from build123d import *

# Parameters (mm, degrees)
F0_R         = 12.5
F1_DEPTH     = 3
F2_R         = 4
F3_DEPTH     = 30
F4_W         = 68
F4_H         = 8
F5_DEPTH     = 8
F6_R         = 3.9999
F7_T8_DEPTH  = 60
F7_S9_R      = 4
F7_T10_DEPTH = 32
F7_S11_R     = 4
F7_T12_DEPTH = 32
F7_T16_DEPTH = 60
F7_S17_R     = 4
F7_T18_DEPTH = 32
F7_S19_R     = 4
F7_T20_DEPTH = 32


# Not quite as in the source:
# - a fillet or chamfer that OpenCascade refuses, or shapes differently, is made with other operations: its cross-section is extruded or revolved along the edge and cut away or added
# - two fillets or chamfers of one size are made in one step
# - a fillet or chamfer is up to 0.001 mm smaller than in the source, because OpenCascade refuses the exact size


with BuildPart() as f1:
    # F0 (on Top) → F1 (new body)
    with BuildSketch(Plane.XY):
        with Locations((-30, 0)):
            Circle(F0_R)
    extrude(amount=F1_DEPTH)

    # F2 (on face) → F3 (join)
    with BuildSketch(Plane.XY.offset(3)):
        with Locations((-30, 0)):
            Circle(F2_R)
    extrude(amount=F3_DEPTH)



with BuildPart() as f1b:
    # F0 (on Top) → F1, piece 2 (new body)
    with BuildSketch(Plane.XY):
        with Locations((30, 0)):
            Circle(F0_R)
    extrude(amount=F1_DEPTH)

    # F2 (on face) → F3, piece 2 (join)
    with BuildSketch(Plane.XY.offset(3)):
        with Locations((30, 0)):
            Circle(F2_R)
    extrude(amount=F3_DEPTH)


with BuildPart() as f1_1:
    add(f1.part)

    add(f1b.part)  # F5 merges F1b
    # F4 (on face) → F5 (join)
    with BuildSketch(Plane.XY.offset(33)):
        Rectangle(F4_W, F4_H)
    extrude(amount=-F5_DEPTH)

    # F6 (radius 4 in the source; OpenCascade refuses exactly that, so slightly less here)
    f6_edges = [f1_1.edges().sort_by_distance(p)[0] for p in [
        (34, 0, 33),
        (0, 4, 33),
        (-34, 0, 33),
        (0, -4, 33),
        (34, -4, 29),
        (34, 4, 29),
        (-34, -4, 29),
        (-34, 4, 29),
    ]]
    fillet(f6_edges, radius=F6_R)

    # F7: fillet of radius 3 on 6 edges, made by hand

    # F7_s1 → F7_t2 (revolve)
    with BuildSketch(Plane.XZ):
        with BuildLine():
            ThreePointArc((33.9996, 6.0009656854), (34.8786796564, 3.8786796564), (37.0009656854, 2.9996))
            Line((37.0009656854, 2.9996), (37.0009656854, 2.6994634315))
            ThreePointArc((37.0009656854, 2.6994634315), (35.5004828427, 2.6998634315), (34, 2.6998634315))
            Line((34, 2.6998634315), (33.6998634315, 3))
            ThreePointArc((33.6998634315, 3), (33.6998634315, 4.5004828427), (33.6994634315, 6.0009656854))
            Line((33.6994634315, 6.0009656854), (33.9996, 6.0009656854))
        make_face()
    revolve(axis=Axis((30, 0, 3), (0, 0, 1)))

    # F7_s3 → F7_t4 (revolve)
    with BuildSketch(Plane.XZ):
        with BuildLine():
            ThreePointArc((-26.0004, 6.0009656854), (-25.1213203436, 3.8786796564), (-22.9990343146, 2.9996))
            Line((-22.9990343146, 2.9996), (-22.9990343146, 2.6994634315))
            ThreePointArc((-22.9990343146, 2.6994634315), (-24.4995171573, 2.6998634315), (-26, 2.6998634315))
            Line((-26, 2.6998634315), (-26.3001365685, 3))
            ThreePointArc((-26.3001365685, 3), (-26.3001365685, 4.5004828427), (-26.3005365685, 6.0009656854))
            Line((-26.3005365685, 6.0009656854), (-26.0004, 6.0009656854))
        make_face()
    revolve(axis=Axis((-30, 0, 3), (0, 0, 1)))


with BuildPart() as f7_tool6:
    # F7_s7 → F7_t8 (new body)
    with BuildSketch(Plane.YZ.offset(-30)):
        with BuildLine():
            ThreePointArc((-0.9990343146, 24.9996), (-3.1213203436, 25.8786796564), (-4.0004, 28.0009656854))
            Line((-4.0004, 28.0009656854), (-4.3005365685, 28.0009656854))
            ThreePointArc((-4.3005365685, 28.0009656854), (-4.3001365685, 26.5004828427), (-4.3001365685, 25))
            Line((-4.3001365685, 25), (-4, 24.6998634315))
            ThreePointArc((-4, 24.6998634315), (-2.4995171573, 24.6998634315), (-0.9990343146, 24.6994634315))
            Line((-0.9990343146, 24.6994634315), (-0.9990343146, 24.9996))
        make_face()
    extrude(amount=F7_T8_DEPTH)

    # F7_s9 → F7_t10 (cut, symmetric)
    with BuildSketch(Plane.XY.offset(26.4)):
        with Locations((30, 0)):
            Circle(F7_S9_R)
    extrude(amount=F7_T10_DEPTH, both=True, mode=Mode.SUBTRACT)

    # F7_s11 → F7_t12 (cut, symmetric)
    with BuildSketch(Plane.XY.offset(26.4)):
        with Locations((-30, 0)):
            Circle(F7_S11_R)
    extrude(amount=F7_T12_DEPTH, both=True, mode=Mode.SUBTRACT)


with BuildPart() as f1_2:
    add(f1_1.part)

    # F7_t5: cut F7_tool6
    add(f7_tool6.part, mode=Mode.SUBTRACT)


with BuildPart() as f7_tool14:
    # F7_s15 → F7_t16 (new body)
    with BuildSketch(Plane.YZ.offset(30)):
        with BuildLine():
            ThreePointArc((4.0004, 28.0009656854), (3.1213203436, 25.8786796564), (0.9990343146, 24.9996))
            Line((0.9990343146, 24.9996), (0.9990343146, 24.6994634315))
            ThreePointArc((0.9990343146, 24.6994634315), (2.4995171573, 24.6998634315), (4, 24.6998634315))
            Line((4, 24.6998634315), (4.3001365685, 25))
            ThreePointArc((4.3001365685, 25), (4.3001365685, 26.5004828427), (4.3005365685, 28.0009656854))
            Line((4.3005365685, 28.0009656854), (4.0004, 28.0009656854))
        make_face()
    extrude(amount=-F7_T16_DEPTH)

    # F7_s17 → F7_t18 (cut, symmetric)
    with BuildSketch(Plane.XY.offset(26.4)):
        with Locations((30, 0)):
            Circle(F7_S17_R)
    extrude(amount=F7_T18_DEPTH, both=True, mode=Mode.SUBTRACT)

    # F7_s19 → F7_t20 (cut, symmetric)
    with BuildSketch(Plane.XY.offset(26.4)):
        with Locations((-30, 0)):
            Circle(F7_S19_R)
    extrude(amount=F7_T20_DEPTH, both=True, mode=Mode.SUBTRACT)


with BuildPart() as f1_3:
    add(f1_2.part)

    # F7_t13: cut F7_tool14
    add(f7_tool14.part, mode=Mode.SUBTRACT)

    # F7_s21 → F7_t22 (revolve, cut)
    with BuildSketch(Plane.XZ):
        with BuildLine():
            ThreePointArc((39.4990343146, 3.0004), (41.6213203436, 2.1213203436), (42.5004, -0.0009656854))
            Line((42.5004, -0.0009656854), (42.8005365685, -0.0009656854))
            ThreePointArc((42.8005365685, -0.0009656854), (42.8001365685, 1.4995171573), (42.8001365685, 3))
            Line((42.8001365685, 3), (42.5, 3.3001365685))
            ThreePointArc((42.5, 3.3001365685), (40.9995171573, 3.3001365685), (39.4990343146, 3.3005365685))
            Line((39.4990343146, 3.3005365685), (39.4990343146, 3.0004))
        make_face()
    revolve(axis=Axis((30, 0, 3), (0, 0, 1)), mode=Mode.SUBTRACT)

    # F7_s23 → F7_t24 (revolve, cut)
    with BuildSketch(Plane.XZ):
        with BuildLine():
            ThreePointArc((-20.5009656854, 3.0004), (-18.3786796564, 2.1213203436), (-17.4996, -0.0009656854))
            Line((-17.4996, -0.0009656854), (-17.1994634315, -0.0009656854))
            ThreePointArc((-17.1994634315, -0.0009656854), (-17.1998634315, 1.4995171573), (-17.1998634315, 3))
            Line((-17.1998634315, 3), (-17.5, 3.3001365685))
            ThreePointArc((-17.5, 3.3001365685), (-19.0004828427, 3.3001365685), (-20.5009656854, 3.3005365685))
            Line((-20.5009656854, 3.3005365685), (-20.5009656854, 3.0004))
        make_face()
    revolve(axis=Axis((-30, 0, 3), (0, 0, 1)), mode=Mode.SUBTRACT)


solid = f1_3.part
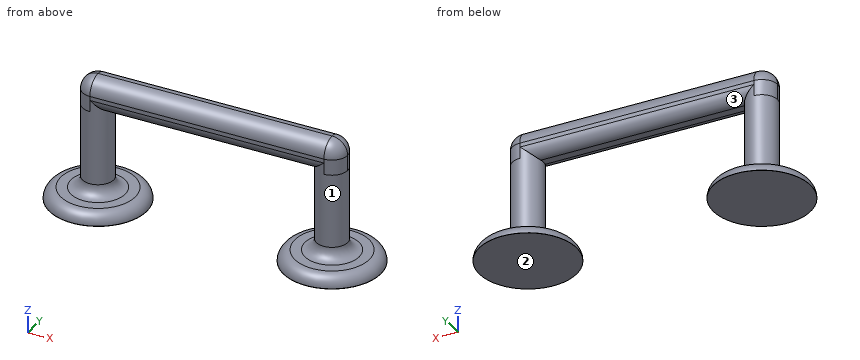
Build history of the part. All positions in model axes, mm. Face numbers are marked on the shaded views. A direction names the side the tool comes from. Round coordinates to 2 decimals unless told otherwise and drop trailing zeros. Loops run counter-clockwise (first coordinate to the right, second up) from the corner with the lowest first, then second, coordinate; pieces in that order, holes last. Notation, with made-up numbers: (66.25, 83) -> (111.25, 83) arc R15 ccw to (111.25, 99) -> close; hole circle Ø8 at (17.25, 32.5). An arc over 180 degrees is marked (long way). One line per item, written item: value. Start each with the question number.
Q1. Drop flat-ended pins along their axis: pin 1 Ø1.5 at (x, y) = (25, 2.5) entering from +Z; pin 2 Ø1.2 at (x, z) = (10, 27) entering from -Y; pin 3 Ø3 at (x, y) = (-23.5, 3.5) entering from -Z; pin 4 Ø2 at (x, y) = (-10, 2) entering from -Z. Give the stop position or say it passes through.
Q2. 3-axis set-ups, long thin cutter, end or side, ignore diameter. For the marked faces 1, 2 and 3: which of +Z, -Z, +X, -X, +Y, -Y reach the whole face in a straight line?
Q3. Cut at D-D on z = 5. List the corners of the cut face in (x, y), plus the area to 3 significant figures.
Q4. Probe line 1 along X through (y, z) = (0.25, 12); line 2 along Z through (x, y) = (37.5, -6); line 3 along Z through (x, y) = (-22, -0.75). List the from-to ranges inside material, lowest first.
Q5. Cut at B-B on z = 10.5. List the corners of the cut face in (x, y).
Computed:
1. pin 1: z = 32.6
1. pin 2: y = -3.97
1. pin 3: z = 0
1. pin 4: z = 25
2. face 1: none
2. face 2: -Z, +X, -X, +Y, -Y
2. face 3: +Y
3. outline: circle Ø8.34 at (-30, 0); circle Ø8.34 at (30, 0)
3. area: 109 mm²
4. line 1: -33.99 to -26.01, 26.01 to 33.99
4. line 2: 0 to 3
4. line 3: 0 to 3, 25 to 32.93
5. outline: circle Ø8 at (-30, 0); circle Ø8 at (30, 0)
